The listing builds one solid part. Answer for the finished solid, in the listing's coordinates (mm). Coordinates: 2 decimals unless noted, no trailing zeros. Loops run counter-clockwise (first coordinate to the right, second up) from the corner with the lowest first, then second, coordinate; pieces in that order, holes last. Notation, with made-up numbers: (53, -22) - (59, -22) arc R27 cw to (59, -6) - close; hole circle Ø3 at (23.5, -35.5). An arc over 180 degrees is marked (long way). One line per question, with ' | ' between items.
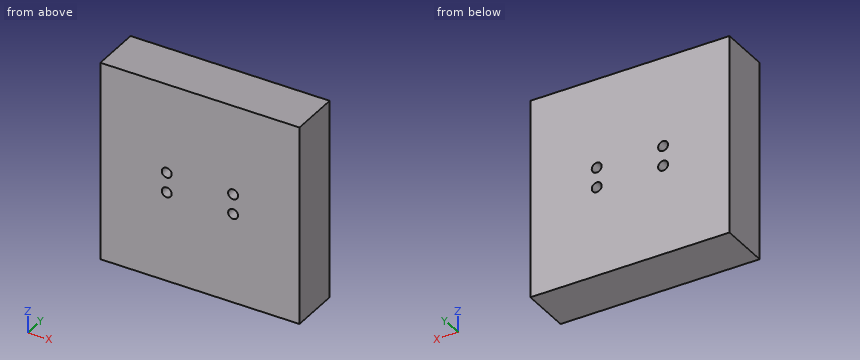
Autodesk Inventor part; units mm, degrees
ref_plane "YZ Plane" through (0, 0, 0) normal (1, 0, 0) x (0, 1, 0)
ref_plane "XZ Plane" through (0, 0, 0) normal (0, 1, 0) x (-1, 0, 0)
ref_plane "XY Plane" through (0, 0, 0) normal (0, 0, 1) x (1, 0, 0)
sketch "Sketch1" plane through (0, 0, 0) normal (0, 1, 0) x (-1, 0, 0)
  line L0 (0, 0) -> (-25.4, 0)
  line L1 (-25.4, 0) -> (-25.4, -25.4)
  line L2 (-25.4, -25.4) -> (0, -25.4)
  line L3 (0, -25.4) -> (0, 0)
  dimension "d0" = 25.4
extrude "Extrusion1" add sketch "Sketch1" along normal blind 6.35
sketch "Sketch2" plane through (0, 6.35, 0) normal (0, 1, 0) x (1, 0, 0)
  circle A0 centre (8.4667, 13.97) radius 0.635
  circle A1 centre (16.9333, 13.97) radius 0.635
  circle A2 centre (16.9333, 11.43) radius 0.635
  circle A3 centre (8.4667, 11.43) radius 0.635
  line L0 (25.4, 0) -> (25.4, 25.4)
  line L1 (0, 0) -> (25.4, 0)
  dimension "d3" = 8.4667
  dimension "d4" = 8.4667
  dimension "d5" = 2.54
  dimension "d6" = 1.27
  dimension "d7" = 11.43
extrude "Extrusion2" cut sketch "Sketch2" against normal blind 6.35
equation "\"d1\" = 0.25 * d0"
equation "\"d3\" = 0.333333 * d0"
equation "\"d4\" = d3"
equation "\"d8\" = 0.25 * d0"
properties part number "pieceBase"
Item 1: Find the intervals of material crossed by line 1 (X direction, y = 4.5, z = -11.43); line 2 (Z direction, x = 8.5, y = 4), in increasing order. Write a range as [from, to].
Taken from the geometry:
line 1: x = [0, 7.83], [9.1, 16.3], [17.57, 25.4] | line 2: z = [-25.4, -14.6], [-13.34, -12.06], [-10.8, 0]
Item 2: Each of these flat-tipped pins is pushed along its axis until it touches: pin 1 Ø1.7 at (x, z) = (8.47, -11.43) entering from +Y; pin 2 Ø0.8 at (x, z) = (8.47, -13.97) entering from +Y. Where does it stop, or does it pass through?
Taken from the geometry:
pin 1: stops at y = 6.35 | pin 2: passes through
Item 3: Find section A-A, the plane z = -13.97. Write down the section's boundary in (x, y), plus the area to 3 significant figures.
Taken from the geometry:
outline: (0, 0) - (7.83, 0) - (7.83, 6.35) - (0, 6.35) - close; (9.1, 0) - (16.3, 0) - (16.3, 6.35) - (9.1, 6.35) - close; (17.57, 0) - (25.4, 0) - (25.4, 6.35) - (17.57, 6.35) - close | area: 145 mm2
Item 4: Find section B-B, the plane x = 8.75. Write down the section's boundary in (y, z), plus the area to 3 significant figures.
Taken from the geometry:
outline: (0, -25.4) - (6.35, -25.4) - (6.35, -14.54) - (0, -14.54) - close; (0, -13.4) - (6.35, -13.4) - (6.35, -12) - (0, -12) - close; (0, -10.86) - (6.35, -10.86) - (6.35, 0) - (0, 0) - close | area: 147 mm2
